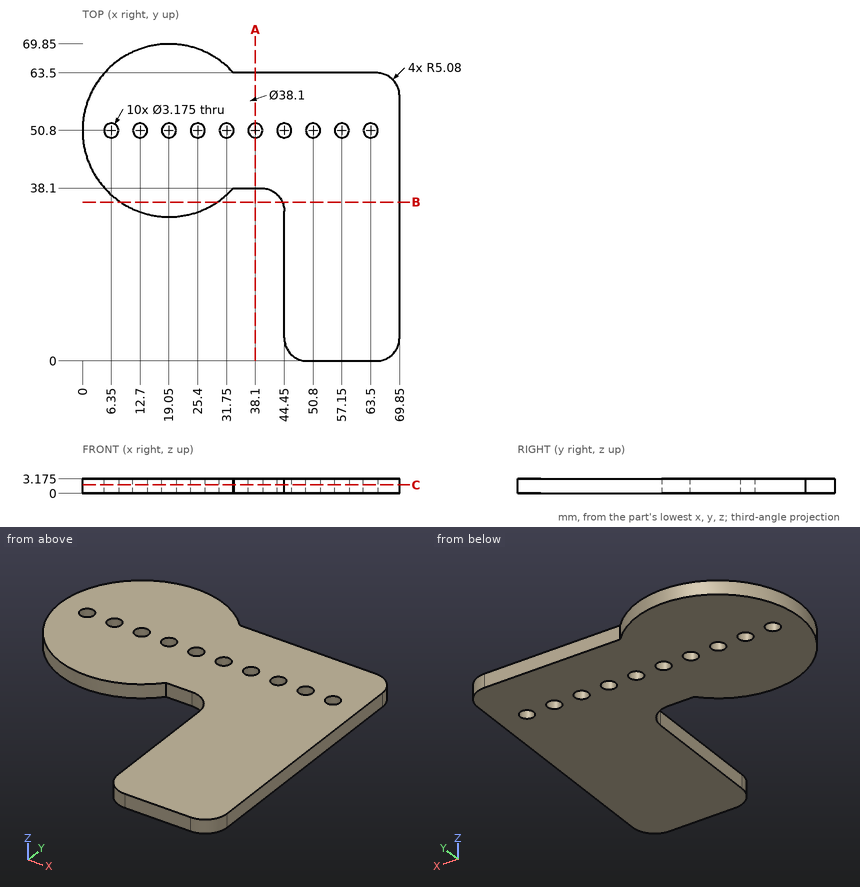
Here's the drawing with two shaded views (mm, measured from the low corner). I have some questions. Give positions to 0.01 mm unless a question says otherwise; leave off trailing zeros. Loops run counter-clockwise (first coordinate to the right, second up) from the corner with the lowest first, then second, coordinate; pieces in that order, holes last. Notation, with made-up numbers: (67.5, 54.5) - (97.5, 54.5) arc R20 ccw to (97.5, 81.5) - close; hole circle Ø2 at (60.5, 82.5). An arc over 180 degrees is marked (long way). Answer in a Markdown table with one row per item. Add a question column.
Q1. If we section it at A-A (x = 38.1): List the corners of the cut face in (y, z) for me (1 decimal).
Q2. For pin 1 (1.9 mm diameter, centred on x = 19.05, y = 50.8, fed in from -Z); pin 2 (8 mm diameter, centred on x = 41.5, y = 16, fed in from -Z); pin 3 (1 mm diameter, centred on x = 47, z = 2.5, fed in from +Y); pin 4 (1.5 mm diameter, centred on y = 57.5, z = 0.5, fed in from -X), each with a flat end and sliding along its axis, tell me the tip position at first contact or that it passes through.
Q3. Please list where these lines run through material, in increasing order: L1, parallel to Y at x = 57.15, z = 1.1; L2, parallel to X at y = 17, z = 1.7; L3, parallel to Y at x = 36, z = 1.25. Write a range as from..to.
Q4. If we section it at B-B (y = 35): List the corners of the cut face in (x, z) for me (3 decimals).
Q5. If we section it at C-C (z = 1.9): State how many separate pieces and enclosed holes the cut face has, plus the area to 3 significant figures.
The answers:
| question | item | result |
|---|---|---|
| 1 | outline | (38.1, 0) - (49.2, 0) - (49.2, 3.2) - (38.1, 3.2) - close; (52.4, 0) - (63.5, 0) - (63.5, 3.2) - (52.4, 3.2) - close |
| 2 | pin 1 | passes through |
| 2 | pin 2 | stops at z = 0 |
| 2 | pin 3 | stops at y = 63.5 |
| 2 | pin 4 | stops at x = 0.95 |
| 3 | L1 | y = 0..49.21, 52.39..63.5 |
| 3 | L2 | x = 44.45..69.85 |
| 3 | L3 | y = 38.1..63.5 |
| 4 | outline | (8.408, 0) - (29.692, 0) - (29.692, 3.175) - (8.408, 3.175) - close; (44.048, 0) - (69.85, 0) - (69.85, 3.175) - (44.048, 3.175) - close |
| 5 | separate pieces | 1 |
| 5 | enclosed holes | 10 |
| 5 | area | 2,860 mm^2 |
